Autodesk Inventor part; units mm, degrees
ref_plane "Work Plane1" through (-30, 0, 20) normal (0, 0, 1) x (1, 0, 0)
ref_plane "YZ Plane" through (0, 0, 0) normal (1, 0, 0) x (0, 1, 0)
ref_plane "XZ Plane" through (0, 0, 0) normal (0, 1, 0) x (-1, 0, 0)
sketch "Sketch1" plane through (0, 0, 0) normal (0, 1, 0) x (-1, 0, 0)
  line L0 (0, 0) -> (34, 0)
  line L1 (34, 0) -> (34, -34)
  line L2 (34, -34) -> (0, -34)
  line L3 (0, -34) -> (0, 0)
  dimension "d0" = 34
  dimension "d1" = 34
extrude "Extrusion1" add sketch "Sketch1" along normal blind 54
sketch "Sketch4" plane through (0, 54, 0) normal (0, 1, 0) x (1, 0, 0)
  point P0 (0, 0)
sketch "Sketch5" plane through (0, 54, 0) normal (0, 1, 0) x (1, 0, 0)
  line L0 (-34, 34) -> (-34, 0)
  line L1 (0, 0) -> (-34, 0)
  line L2 (-34, 0) -> (-34, 34)
  line L3 (-34, 34) -> (0, 34)
  line L4 (0, 34) -> (0, 0)
  line L5 (4, 38) -> (-38, 38)
  line L6 (-38, 38) -> (-38, -4)
  line L7 (-38, -4) -> (4, -4)
  line L8 (4, -4) -> (4, 38)
  dimension "d15" = 4
extrude "Extrusion2" add sketch "Sketch5" along normal blind 5 contours L3 L4 L1 L0 | L8 L7 L6 L5
sketch "Sketch6" plane through (0, 59, 0) normal (0, 1, 0) x (1, 0, 0)
  line L0 (-34, 34) -> (-34, 0)
  circle A0 centre (-34, 34) radius 2
  line L1 (-38, 38) -> (-38, -4)
  line L2 (-38, 38) -> (-38, 34)
  line L3 (-38, 38) -> (-34, 38)
  line L4 (4, 38) -> (-38, 38)
  circle A1 centre (-34, 0) radius 2
  circle A2 centre (0, 34) radius 2
  circle A3 centre (0, 0) radius 2
  point P0 (0, 0)
  dimension "d18" = 4
  dimension "d21" = 34
  dimension "d24" = 34
extrude "Extrusion3" cut sketch "Sketch6" against normal blind 5
sketch "Sketch8" plane through (0, 0, 0) normal (0, -1, 0) x (1, 0, 0)
  line L0 (0, -32) -> (0, -34)
  line L1 (0, -2) -> (0, -32)
  arc A0 (0, -30) -> (-4, -34) centre (0, -34) ccw
  line L2 (-32, -34) -> (-34, -34)
  line L3 (-34, -32) -> (-34, -2)
  line L4 (-34, -34) -> (-30, -34) construction
  line L5 (-34, -34) -> (-30, -34) construction
  line L6 (0, -34) -> (-4, -34)
  line L7 (-2, -34) -> (-32, -34)
  line L8 (0, -30) -> (0, -34)
  line L9 (-17, -34) -> (-17, -17)
  circle A1 centre (-17, -17) radius 1.5
  arc A2 (-4, 0) -> (0, -4) centre (0, 0) ccw
  line L10 (0, 0) -> (0, -4)
  line L11 (-4, 0) -> (0, 0)
  arc A3 (-34, -4) -> (-30, 0) centre (-34, 0) ccw
  line L12 (-34, 0) -> (-30, 0)
  line L13 (-34, -4) -> (-34, 0)
  arc A4 (-30, -34) -> (-34, -30) centre (-34, -34) ccw
  line L14 (-34, -34) -> (-34, -30)
  line L15 (-30, -34) -> (-34, -34)
  point P0 (0, 0)
  point P1 (0, -2)
  point P2 (-2, 0)
  point P3 (-32, 0)
  point P4 (-34, -2)
  point P5 (-34, -32)
  point P6 (-32, -34)
  dimension "d29" = 4
  dimension "d31" = 0
  dimension "d32" = 3
  dimension "d33" = 17
  dimension "d36" = 360
extrude "Extrusion4" cut sketch "Sketch8" against normal up to surface (54 mm away) contours L3 L13 L12 A3 | L7 L2 L14 L3 A4 | A2 L11 L10 L1 | L0 L6 A0 L1
sketch "Sketch9" plane through (0, 59, 0) normal (0, 1, 0) x (1, 0, 0)
  line L0 (-38, -4) -> (4, -4)
  line L1 (-17, -4) -> (-17, 17)
  circle A0 centre (-17, 17) radius 15
  point P0 (0, 0)
  dimension "d40" = 21
  dimension "d41" = 30
extrude "Extrusion5" add sketch "Sketch9" along normal blind 1
sketch "Sketch10" plane through (-17, 60, -17) normal (0, 1, 0) x (1, 0, 0)
  circle A0 centre (0, 0) radius 15
  circle A1 centre (0, 0) radius 4
  line L0 (0, 0) -> (0, 3.75)
  line L1 (0, 3.75) -> (1.3919, 3.75)
  line L2 (0, 3.75) -> (-1.3919, 3.75)
  point P0 (17, -17)
  dimension "d44" = 8
  dimension "d45" = 3.75
extrude "Extrusion6" add sketch "Sketch10" along normal blind 15 contours A1 L2 L1 picked at (-0.0068, -1.3972)
fillet "Fillet1" radius 4 4 edges at (4, 56.5, -38) (4, 56.5, 4) (-38, 56.5, -38) (-38, 56.5, 4)
sketch "Sketch11" plane through (-30, 0, 0) normal (0, 0, 1) x (1, 0, 0)
  line L0 (26, 0) -> (0, 0)
  line L1 (13, 0) -> (13, 17)
  line L2 (6.5, 27) -> (19.5, 27)
  line L3 (19.5, 27) -> (19.5, 7)
  line L4 (19.5, 7) -> (6.5, 7)
  line L5 (6.5, 7) -> (6.5, 27)
  line L6 (6.5, 27) -> (19.5, 7) construction
  line L7 (19.5, 27) -> (6.5, 7) construction
  point P0 (30, 0)
  dimension "d49" = 17
  dimension "d50" = 13
  dimension "d51" = 20
extrude "Extrusion7" add sketch "Sketch11" along normal blind 5
ref_plane "Work Plane1" through (-30, 0, 20) normal (0, 0, 1) x (1, 0, 0)
sketch "Sketch12" plane through (-30, 0, 20) normal (0, 0, 1) x (1, 0, 0)
  line L0 (6.5, 7) -> (6.5, 27)
  line L1 (6.5, 7) -> (6.5, 0)
  line L2 (26, 0) -> (0, 0)
  circle A0 centre (6.5, 0) radius 4
  line L3 (19.5, 7) -> (6.5, 7)
  line L4 (19.5, 7) -> (19.5, 0)
  circle A1 centre (19.5, 0) radius 4
  point P0 (30, 0)
  dimension "d61" = 8
  dimension "d62" = 8
sketch "Sketch13" plane through (0, 0, 0) normal (0, -1, 0) x (1, 0, 0)
  line L0 (0, -30) -> (0, -4)
  line L1 (0, -17) -> (-17, -17)
  circle A0 centre (-17, -17) radius 15
  point P0 (0, 0)
  dimension "d57" = 17
  dimension "d58" = 30
extrude "Extrusion8" add sketch "Sketch13" along normal blind 12
sketch "Sketch14" plane through (-23.5, 7, 0) normal (0, -1, 0) x (1, 0, 0)
  point P0 (23.5, 0)
sketch "Sketch15" plane through (-30, 0, 5) normal (0, 0, 1) x (1, 0, 0)
  line L0 (6.5, 7) -> (6.5, 27)
  line L1 (6.5, 17) -> (13, 17)
  circle A0 centre (13, 17) radius 4
  line L2 (13, 17) -> (13, -6)
  circle A1 centre (13, -6) radius 4
  point P0 (30, 0)
  dimension "d63" = 6.5
  dimension "d64" = 8
  dimension "d65" = 23
  dimension "d66" = 8
extrude "Extrusion9" add sketch "Sketch15" along normal mid plane 20
properties part number "NEMA17_Stepper_CL42H60"
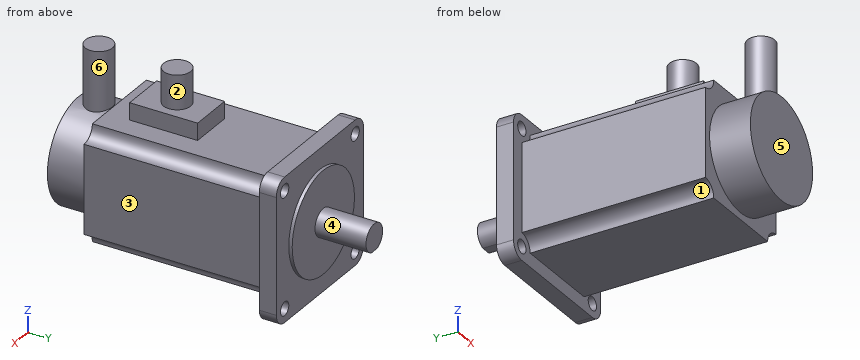
Part model, mm, in its own coordinate system. Face numbers are marked on the shaded views. A direction names the side the tool comes from. Coordinates: 2 decimals unless noted, no trailing zeros. Loops run counter-clockwise (first coordinate to the right, second up) from the corner with the lowest first, then second, coordinate; pieces in that order, holes last. Notation, with made-up numbers: (-10, 3) -> (12, 3) arc R19 cw to (12, 11) -> close; hole circle Ø8 at (5.25, -6.75). An arc over 180 degrees is marked (long way). Use a Markdown table: item, result. Add a question column.
Item 1: Band-saw the part on C-C on z = 6. Write the cut outline in (x, y), plus the area to 3 significant figures.
Item 2: Band-saw the part on B-B on z = -17. Write the cut outline in (x, y).
Item 3: Flat gauge pins, fed straight in: P1, Ø10, axis at x = -8, y = 64.5, coming from the +Z side; P2, Ø4.5, axis at x = 0, z = 0, coming from the +Y side; P3, Ø12, axis at y = 22.5, z = -15, coming from the -X side; P4, Ø1, axis at x = -26.5, y = 62, coming from the +Z side. Where does each tip first touch, or does it go through?
Item 4: Which spindle directions (+Z, -Z, +X, -X, +Y, -Y) get a long thin tool onto all of the face, cutting with end or side? Do the marked faces 1, 2 and 3. Say none if no direction does.
Item 5: Pull direction Y, two halves, no side cores. Call the marked faces 4, 5 and 6: +Y half, -Y half, draft (parallel to the pull), parting line (faces both ways), or undercut.
Item 6: Probe probe 1 along X at (y, z) = (57, 0); probe 2 along Y at (x, z) = (-2.5, -27.5). List the from-to ranges inside material, lowest first.
Item 7: Band-saw the part on D-D on y = 17. Write the cut outline in (x, z).
Geometry says:
| question | item | result |
|---|---|---|
| 1 | outline | circle Ø8 at (-17, -6); circle Ø8 at (-17, 17) |
| 1 | area | 101 mm² |
| 2 | outline | (-38, 54) -> (-34, 54) -> (-34, 0) -> (-32, 0) -> (-32, -12) -> (-2, -12) -> (-2, 0) -> (0, 0) -> (0, 54) -> (4, 54) -> (4, 59) -> (-2, 59) -> (-2, 60) -> (-13, 60) -> (-13, 75) -> (-21, 75) -> (-21, 60) -> (-32, 60) -> (-32, 59) -> (-38, 59) -> close |
| 3 | P1 | z = -3.64 |
| 3 | P2 | y = 59 |
| 3 | P3 | x = -34 |
| 3 | P4 | through |
| 4 | face 1 | -Z, -X, -Y |
| 4 | face 2 | +Z |
| 4 | face 3 | +Z, -Z, +X, -Y |
| 5 | face 4 | draft |
| 5 | face 5 | -Y half |
| 5 | face 6 | undercut |
| 6 | probe 1 | -38 to -36, -32 to -2, 2 to 4 |
| 6 | probe 2 | 0 to 59 |
| 7 | outline | (-34, -30) arc R4 cw to (-30, -34) -> (-4, -34) arc R4 cw to (0, -30) -> (0, -4) arc R4 cw to (-4, 0) -> (-10.5, 0) -> (-10.5, 5) -> (-13, 5) -> (-13, 15) -> (-21, 15) -> (-21, 5) -> (-23.5, 5) -> (-23.5, 0) -> (-30, 0) arc R4 cw to (-34, -4) -> close |
